Read the model definition and answer for the solid it produces. Units are mm, in the model's axes. Face numbers are marked on the shaded views. Coordinates: 2 decimals unless noted, no trailing zeros. Loops run counter-clockwise (first coordinate to the right, second up) from the corner with the lowest first, then second, coordinate; pieces in that order, holes last. Notation, with made-up numbers: (2, -0.75) -> (17, -0.75) arc R7 ccw to (17, 7.25) -> close; hole circle Ø3 at (56.5, 24). An arc over 180 degrees is marked (long way). Answer as a JSON object with one key per item and string values. Group by question number.
1) Section D-D, the plane z = 4.75 is taken. Count the separate pieces of the cut face and the enclosed holes in it, plus the area to 3 significant figures.
2) A flat-ended cylindrical pin translates along its axis: P1, Ø2.5, axis at x = 14, y = 11, coming from the +Z side. Find the tip coordinate at first contact, or state that the pin passes through.
3) Section B-B, the plane x = 14 is taken. Give the vertices of the cut face in (y, z) (3 decimals).
4) Consider probe 1 along X at (y, z) = (4, 4) (3 decimals); probe 2 along Y at (x, z) = (14, 1.5) (3 decimals). Determine where each line is inside the solid, lowest interval first. Write a range as [from, to].
5) Determine the mould class of the marked faces 1, 2, 3 and 4 for opening direction Y: released by +Y, released by -Y, zero draft, split by the parting line, or undercut.
6) Section C-C, the plane y = 4 is taken. Give the vertices of the cut face in (x, z) (3 decimals).
7) Section A-A, the plane y = 18 is taken. Give the vertices of the cut face in (x, z) (3 decimals).
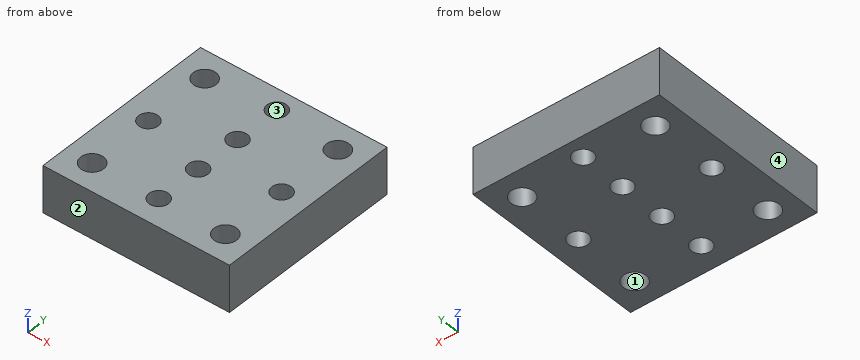
Autodesk Fusion 360 part; units mm, degrees
sketch "Sketch1" plane through (0, 0, 0) normal (0, 0, 1) x (1, 0, 0)
  line L0 (0, 28) -> (28, 28)
  line L1 (28, 28) -> (28, 0)
  line L2 (28, 0) -> (0, 0)
  line L3 (0, 0) -> (0, 28)
  dimension "d1" = 28
  dimension "d2" = 28
  dimension "d13" = 28
  dimension "d14" = 28
sketch "Sketch2" plane through (0, 0, 0) normal (0, 0, 1) x (1, 0, 0)
  circle A0 centre (4, 24) radius 1.5
  circle A1 centre (4, 4) radius 1.5
  circle A2 centre (24, 4) radius 1.5
  circle A3 centre (24, 24) radius 1.5
  circle A4 centre (4, 14) radius 1.5
  circle A5 centre (14, 25) radius 1.5
  circle A6 centre (14, 18) radius 1.5
  circle A7 centre (14, 4) radius 1.5
  circle A8 centre (24, 14) radius 1.5
  circle A9 centre (14, 11) radius 1.5
  dimension "d15" = 3
  dimension "d16" = 3
  dimension "d17" = 3
  dimension "d18" = 3
  dimension "d19" = 3
  dimension "d20" = 3
  dimension "d21" = 3
  dimension "d22" = 3
  dimension "d23" = 3
  dimension "d24" = 3
  dimension "d25" = 10
  dimension "d26" = 10
  dimension "d27" = 10
  dimension "d28" = 10
  dimension "d29" = 10
  dimension "d30" = 10
  dimension "d31" = 7
  dimension "d32" = 7
  dimension "d33" = 7
extrude "Extrude1" add sketch "Sketch1" along normal blind 7
hole "Hole1" at (14, 25, 0) at (4, 14, 0) at (14, 18, 0) at (14, 11, 0) at (24, 14, 0) at (14, 4, 0) direction (0, 0, 1) diameter 2.93 depth 7 tip angle 180
sketch "Sketch3" plane through (0, 0, 7) normal (0, 0, 1) x (-1, 0, 0)
  circle A0 centre (-24, -14) radius 1.465
  circle A1 centre (-14, -18) radius 1.465
  circle A2 centre (-14, -25) radius 1.465
  circle A3 centre (-4, -14) radius 1.465
  circle A4 centre (-14, -11) radius 1.465
  circle A5 centre (-14, -4) radius 1.465
  line L0 (0, 0) -> (-28, 0)
  line L1 (-28, 0) -> (-28, -28)
  line L2 (-28, -28) -> (0, -28)
  line L3 (0, -28) -> (0, 0)
  circle A6 centre (-4, -24) radius 2
  circle A7 centre (-4, -4) radius 2
  circle A8 centre (-24, -4) radius 2
  circle A9 centre (-24, -24) radius 2
hole "Hole2" at (4, 24, 7) at (24, 24, 7) at (24, 4, 7) at (4, 4, 7) direction (0, 0, -1) diameter 3.4 depth 7 tip angle 180
Determined:
{
 "1": {"separate pieces": "1", "enclosed holes": "10", "area": "707 mm²"},
 "2": {"P1": "through"},
 "3": {"outline": "(0, 0) -> (2.535, 0) -> (2.535, 7) -> (0, 7) -> close; (5.465, 0) -> (9.535, 0) -> (9.535, 7) -> (5.465, 7) -> close; (12.465, 0) -> (16.535, 0) -> (16.535, 7) -> (12.465, 7) -> close; (19.465, 0) -> (23.535, 0) -> (23.535, 7) -> (19.465, 7) -> close; (26.465, 0) -> (28, 0) -> (28, 7) -> (26.465, 7) -> close"},
 "4": {"probe 1": "[0, 2.3], [5.7, 12.535], [15.465, 22.3], [25.7, 28]", "probe 2": "[0, 2.535], [5.465, 9.535], [12.465, 16.535], [19.465, 23.535], [26.465, 28]"},
 "5": {"face 1": "undercut", "face 2": "released by -Y", "face 3": "undercut", "face 4": "zero draft"},
 "6": {"outline": "(0, 0) -> (2.3, 0) -> (2.3, 7) -> (0, 7) -> close; (5.7, 0) -> (12.535, 0) -> (12.535, 7) -> (5.7, 7) -> close; (15.465, 0) -> (22.3, 0) -> (22.3, 7) -> (15.465, 7) -> close; (25.7, 0) -> (28, 0) -> (28, 7) -> (25.7, 7) -> close"},
 "7": {"outline": "(0, 0) -> (12.535, 0) -> (12.535, 7) -> (0, 7) -> close; (15.465, 0) -> (28, 0) -> (28, 7) -> (15.465, 7) -> close"}
}
